CAD build for the part. Positions are in the model's coordinates, mm. A direction names the side the tool comes from. Coordinates: 2 decimals unless noted, no trailing zeros. Order: outer loops, then holes, each group sorted by start corner. A loop starts at its lowest first (then second) coordinate and runs counter-clockwise, first axis right, second up. Notation, with made-up numbers: (41, -18) - (60, -18) arc R25 cw to (60, 20) - close; hole circle Ø10 at (12, 86). An arc over 180 degrees is marked (long way). Use one line per item in the form item = value.
```python
from build123d import *

# Parameters (mm, degrees)
SKETCH_1_W             = 8
SKETCH_1_H             = 20
EXTRUDE_1_DEPTH        = 10
SKETCH_2_W             = 5
SKETCH_2_H             = 15
CUT_EXTRUDE_1_DEPTH    = 10
SKETCH_3_W             = 8
SKETCH_3_H             = 5
EXTRUDE_2_DEPTH        = 5
SKETCH_4_W             = 8
SKETCH_4_H             = 5
EXTRUDE_3_DEPTH        = 20
SKETCH_5_W             = 20
SKETCH_5_H             = 30
EXTRUDE_4_DEPTH        = 5
SKETCH_6_R             = 2.5
CUT_EXTRUDE_2_DEPTH    = 5
SKETCH_7_W             = 8
SKETCH_7_H             = 5
EXTRUDE_5_DEPTH        = 15
CUT_EXTRUDE_3_DEPTH    = 10
HOLE_WIZARD_M4_1_D     = 3.3
HOLE_WIZARD_M4_1_DEPTH = 10.1
HOLE_WIZARD_M4_1_TIP   = 0.991420021


with BuildPart() as part:
    # 草图1 → 凸台-拉伸1 (new body)
    with BuildSketch(Plane.XY):
        with Locations((4, 10)):
            Rectangle(SKETCH_1_W, SKETCH_1_H)
    extrude(amount=EXTRUDE_1_DEPTH)

    # 草图2 → 切除-拉伸1 (cut)
    with BuildSketch(Plane.ZY):
        with Locations((2.5, 7.5)):
            Rectangle(SKETCH_2_W, SKETCH_2_H)
    extrude(amount=-CUT_EXTRUDE_1_DEPTH, mode=Mode.SUBTRACT)

    # 草图3 → 凸台-拉伸2 (add)
    with BuildSketch(Plane(origin=(0, 0, 0), x_dir=(-1, 0, 0), z_dir=(0, 0, -1))):
        with Locations((-4, 17.5)):
            Rectangle(SKETCH_3_W, SKETCH_3_H)
    extrude(amount=EXTRUDE_2_DEPTH)

    # 草图4 → 凸台-拉伸3 (add)
    with BuildSketch(Plane.XZ):
        with Locations((4, 7.5)):
            Rectangle(SKETCH_4_W, SKETCH_4_H)
    extrude(amount=EXTRUDE_3_DEPTH)

    # 草图5 → 凸台-拉伸4 (add)
    with BuildSketch(Plane.XZ.offset(20)):
        with Locations((-2, -5)):
            Rectangle(SKETCH_5_W, SKETCH_5_H)
    extrude(amount=EXTRUDE_4_DEPTH)

    # 草图6 → 切除-拉伸2 (cut)
    with BuildSketch(Plane(origin=(0, -20, 0), x_dir=(1, 0, 0), z_dir=(0, 1, 0))):
        with Locations((-4.6, 12.897897411)):
            Circle(SKETCH_6_R)
    extrude(amount=-CUT_EXTRUDE_2_DEPTH, mode=Mode.SUBTRACT)

    # 草图7 → 凸台-拉伸5 (add)
    with BuildSketch(Plane(origin=(0, 0, -5), x_dir=(-1, 0, 0), z_dir=(0, 0, -1))):
        with Locations((-4, 17.5)):
            Rectangle(SKETCH_7_W, SKETCH_7_H)
    extrude(amount=EXTRUDE_5_DEPTH)

    # 草图8 → 切除-拉伸3 (cut)
    with BuildSketch(Plane(origin=(0, 20, 0), x_dir=(1, 0, 0), z_dir=(0, 1, 0))):
        with BuildLine():
            Line((6.25, 14), (6.25, 2))
            ThreePointArc((6.25, 2), (4, -0.25), (1.75, 2))
            Line((1.75, 2), (1.75, 14))
            ThreePointArc((1.75, 14), (4, 16.25), (6.25, 14))
        make_face()
    extrude(amount=-CUT_EXTRUDE_3_DEPTH, mode=Mode.SUBTRACT)

    # M4 螺纹孔1
    with Locations(Plane.XY.offset(10)):
        with Locations((4, 13)):
            Hole(HOLE_WIZARD_M4_1_D / 2, depth=HOLE_WIZARD_M4_1_DEPTH)
            with Locations((0, 0, -(HOLE_WIZARD_M4_1_DEPTH + HOLE_WIZARD_M4_1_TIP / 2))):  # 118° drill point
                Cone(0, HOLE_WIZARD_M4_1_D / 2, HOLE_WIZARD_M4_1_TIP, mode=Mode.SUBTRACT)


solid = part.part
```
Item 1: Cut at D-D, the plane x = 4. Write the cut outline in (y, z).
Derived:
outline = (-25, -20) - (-20, -20) - (-20, 5) - (11.35, 5) - (11.35, 10) - (-25, 10) - close; (14.65, 5) - (15, 5) - (15, 0.25) - (20, 0.25) - (20, 10) - (14.65, 10) - close; (15, -20) - (20, -20) - (20, -16.25) - (15, -16.25) - close
Item 2: Drill centre lines: line 1 (Y direction, x = 1, z = -18); line 2 (Z direction, x = -4.6, y = -22.8); line 3 (Y direction, x = -3, z = 8.75). Where is each one in solid material? Low to high. Write a range as [from, to].
Derived:
line_1 = [-25, -20], [15, 20]
line_2 = [-20, -15.4], [-10.4, 10]
line_3 = [-25, -20]
Item 3: Cut at C-C, the plane z = 7.5. Write the cut outline in (x, y).
Derived:
outline = (-12, -25) - (8, -25) - (8, 20) - (0, 20) - (0, -20) - (-12, -20) - close; hole circle Ø3.3 at (4, 13)
Item 4: Cut at A-A, the plane x = -4.6. Write the cut outline in (y, z).
Derived:
outline = (-25, -20) - (-20, -20) - (-20, -15.4) - (-25, -15.4) - close; (-25, -10.4) - (-20, -10.4) - (-20, 10) - (-25, 10) - close
Item 5: Two-plate mould, pull along Y, no slides. Class faces 1 (the face through (-2, -25, -5)), 2 (the face through (4.05, 17.54, 0.25)), 3 (the face through (1, 15, -7)): +Y half, -Y half, draft (parallel to the pull), parting line (faces both ways), or undercut.
Derived:
face_1 = -Y half
face_2 = draft
face_3 = undercut
Item 6: 3-axis set-ups, long thin cutter, end or side, ignore diameter. For faces 4 (the face through (0, 3, 6)), 5 (the face through (-2, -20, -5)), 6 (the face through (6.25, 18, -8)), 7 (the face through (4, -2, 5)): which of +Z, -Z, +X, -X, +Y, -Y reach the whole face in a straight line?
Derived:
face_4 = +Z, -Z, -X, +Y
face_5 = -Z, -X
face_6 = +Y
face_7 = -Z, +X, -X
Item 7: Drop flat-ended pins along their axis: pin 1 (5.5 mm diameter, centred on y = 16.5, z = -8.5, fed in from -X); pin 2 (6 mm diameter, centred on x = -5.5, y = -9, fed in from -Z); pin 3 (4 mm diameter, centred on x = 6, y = 8.5, fed in from -Z); pin 4 (6 mm diameter, centred on x = -7, z = -10.5, fed in from +Y). Give the stop position or say it passes through.
Derived:
pin_1 = 0
pin_2 = through
pin_3 = 5
pin_4 = -20
Item 8: Cut at B-B, the plane y = 13. Write the cut outline in (x, z), plus the area to 3 significant figures.
Derived:
outline = (0, 5) - (2.35, 5) - (2.35, 10) - (0, 10) - close; (5.65, 5) - (8, 5) - (8, 10) - (5.65, 10) - close
area = 23.5 mm²
